from build123d import *

# Parameters (mm, degrees)
SKETCH_1_R           = 35
SKETCH_1_R_2         = 25
EXTRUDE_1_DEPTH      = 25
SKETCH_2_R           = 1.5
CUT_EXTRUDE_1_DEPTH  = 10
SKETCH_4_R           = 22.5
SKETCH_3_R           = 35
EXTRUDE_2_REACH      = 110.858
EXTRUDE_2_END_RADIUS = 35
SKETCH_7_R           = 6
SKETCH_7_R_2         = 5
SKETCH_9_R           = 6
SKETCH_9_R_2         = 5
EXTRUDE_3_DEPTH      = 20


with BuildPart() as part:
    # 草图1 → 凸台-拉伸1 (new, symmetric)
    with BuildSketch(Plane.XY):
        Circle(SKETCH_1_R)
        Circle(SKETCH_1_R_2, mode=Mode.SUBTRACT)
    extrude(amount=EXTRUDE_1_DEPTH, both=True)

    # 草图2 → 切除-拉伸1 (cut)
    with BuildSketch(Plane(origin=(0, 0, -25), x_dir=(-1, 0, 0), z_dir=(0, 0, -1))):
        with Locations((0, 28.75)):
            Circle(SKETCH_2_R)
        with Locations((28.75, 0)):
            Circle(SKETCH_2_R)
        with Locations((0, -28.75)):
            Circle(SKETCH_2_R)
        with Locations((-28.75, 0)):
            Circle(SKETCH_2_R)
    extrude(amount=-CUT_EXTRUDE_1_DEPTH, mode=Mode.SUBTRACT)

    # 草图4 → Loft 1 section 0
    with BuildSketch(Plane.XY.offset(40)):
        Circle(SKETCH_4_R)
    # 草图3 → Loft 1 section 1
    with BuildSketch(Plane.XY.offset(25)):
        Circle(SKETCH_3_R)
    loft()

    # Loft 1 2: read off the stored shape, not the designer's step
    # Loft 1 2: loft between two sections, ruled curve by curve
    loft_1_2_from = [
        Edge.make_bspline([(-17.413546016, 7.600553608, 37), (-2.212438801, 42.42764564, 37), (32.614653231, 27.226538425, 37), (17.413546016, -7.600553608, 37), (2.212438801, -42.42764564, 37), (-32.614653231, -27.226538425, 37), (-17.413546016, 7.600553608, 37)], [0, 0, 0, 0, 0.5, 0.5, 0.5, 1, 1, 1, 1], 3, [1, 0.333333333, 0.333333333, 1, 0.333333333, 0.333333333, 1]),
    ]
    loft_1_2_to = [
        Edge.make_bspline([(-12.914827658, 21.405775542, 25), (29.896723426, 47.235430858, 25), (55.726378742, 4.423879774, 25), (12.914827658, -21.405775542, 25), (-29.896723426, -47.235430858, 25), (-55.726378742, -4.423879774, 25), (-12.914827658, 21.405775542, 25)], [0, 0, 0, 0, 0.5, 0.5, 0.5, 1, 1, 1, 1], 3, [1, 0.333333333, 0.333333333, 1, 0.333333333, 0.333333333, 1]),
    ]
    loft_1_2 = Solid(Shell([*[Face.make_surface_from_curves(loft_1_2_from[k], loft_1_2_to[k]) for k in range(1)], Face(Wire(loft_1_2_from)), Face(Wire(loft_1_2_to))]))
    add(loft_1_2, mode=Mode.SUBTRACT)

    # 凸台-拉伸2: up to this cylinder (the profile starts outside it)
    extrude_2_end = Plane(origin=(0, 0, -5.830294), z_dir=(0, 0, -1)) * Cylinder(EXTRUDE_2_END_RADIUS, 292.716, mode=Mode.PRIVATE)
    # 草图7 → 凸台-拉伸2 (add, up to the surface)
    with BuildSketch(Plane(origin=(0, 60, 0), x_dir=(1, 0, 0), z_dir=(0, 1, 0)), mode=Mode.PRIVATE) as extrude_2_sk1:
        with Locations(Location((0, 0, 0), (0, 0, 270))):
            Circle(SKETCH_7_R)
        with Locations(Location((0, 0, 0), (0, 0, 270))):
            Circle(SKETCH_7_R_2, mode=Mode.SUBTRACT)
    extrude_2_tool1 = extrude(extrude_2_sk1.sketch, amount=-EXTRUDE_2_REACH, mode=Mode.PRIVATE) - extrude_2_end
    add(extrude_2_tool1.solids().sort_by_distance((0, 60, -5.830294))[0])

    # 草图9 → 凸台-拉伸3 (add)
    with BuildSketch(Plane.XY.offset(60)):
        with Locations((0, 15)):
            Circle(SKETCH_9_R)
        with Locations((0, 15)):
            Circle(SKETCH_9_R_2, mode=Mode.SUBTRACT)
    extrude(amount=-EXTRUDE_3_DEPTH)


solid = part.part
Source: CAD feature listing. Evaluate the final solid. Frame: model axes, mm. A direction names the side the tool comes from. Round coordinates to 2 decimals unless told otherwise and drop trailing zeros. Loops run counter-clockwise (first coordinate to the right, second up) from the corner with the lowest first, then second, coordinate; pieces in that order, holes last. Notation, with made-up numbers: (21, 29) - (76, 29) arc R6 cw to (76, 33) - close; hole circle Ø5 at (-30.5, -27.5). An arc over 180 degrees is marked (long way). Write item = value, one per line. Start each with the question number.
Item 1: Reachability of faces 4 (the face through (-1.08, 10.12, 50.14)), 5 (the face through (0.195, -27.263, -20.07)), 6 (the face through (4, 60, -4)) from +Z, -Z, +X, -X, +Y, -Y: full face, straight path, thin tool, end or side. Return the list, or none.
Item 2: Section query A-A on z = 15. Output: boundary loops of the cut face in (x, y).
Item 3: First-contact query: pin 1 Ø1.5 at (x, y) = (-0.5, -29) entering from -Z; pin 2 Ø3.5 at (x, y) = (0, -28.75) entering from +Z; pin 3 Ø1.8 at (x, y) = (0, 28.75) entering from +Z; pin 4 Ø8 at (x, y) = (-1, 15.5) entering from +Z. Flat tips, straight axial feed; report the tip coordinate or a pass-through.
Item 4: Mould query, pull axis Z, two halves, no side actions, for faces 1 (the face through (30.25, 0.07, -20.07)), 2 (the face through (-4.88, 47.5, -1.08)), 3 (the face through (0, 15, 40)). Classes: released by +Z, released by -Z, zero draft, split by the parting line, or undercut.
Item 5: Material intervals for line 1 (Y direction, x = 0.5, z = 47.5); line 2 (Y direction, x = 0, z = -9); line 3 (Z direction, x = -6, y = 13.5), sorted ascending.
Results list:
q1.face_4 = +Z
q1.face_5 = -Z
q1.face_6 = +Z, -Z, +X, -X, +Y
q2.outline = circle Ø70 at (0, 0); hole circle Ø50 at (0, 0)
q3.pin_1 = -15
q3.pin_2 = 34.6
q3.pin_3 = 33.58
q3.pin_4 = 60
q4.face_1 = zero draft
q4.face_2 = undercut
q4.face_3 = released by +Z
q5.line_1 = 9.02 to 10.03, 19.97 to 20.98
q5.line_2 = -35 to -25, 25 to 35
q5.line_3 = 37 to 40
